Input: dimensioned drawing with shaded views. Units: mm. Origin: part minimum x, y, z. Round coordinates to 2 decimals unless told otherwise and drop trailing zeros. Order: outer loops, then holes, each group sorted by start corner. A loop starts at its lowest first (then second) coordinate and runs counter-clockwise, first axis right, second up. Notation, with made-up numbers: (33.25, 87) - (68.25, 87) arc R31 ccw to (68.25, 122) - close; hole circle Ø3 at (81.5, -8.5). An arc over 180 degrees is marked (long way). Put each result on its own line as item: value. Start each with the question number.
(1) Material intervals for L1, parallel to Y at x = 12, z = 2; L2, parallel to X at y = 38, z = 4.5; L3, parallel to Y at x = 24, z = 2.25, sorted ascending. Write a range as [from, to].
(2) Section C-C (z = 3.35). Output: boundary loops of the cut face in (x, y).
(3) Section A-A (y = 42). Output: boundary loops of the cut face in (x, z), and give its area (3 significant figures).
(4) Section B-B (x = 12). Output: boundary loops of the cut face in (y, z).
(5) Section D-D (x = 84). Output: boundary loops of the cut face in (y, z).
(6) Pin query (flat end, axial travel): P1, Ø1.3, axis at y = 2.5, z = 2, coming from the +X side; P2, Ø3.5, axis at x = 15, y = 74, coming from the +Z side; P3, Ø1.3, axis at y = 78.5, z = 4, coming from the +X side; P4, Ø1, axis at x = 68, z = 1.5, coming from the +Y side. Return the tip coordinate at first contact, or that it passes through.
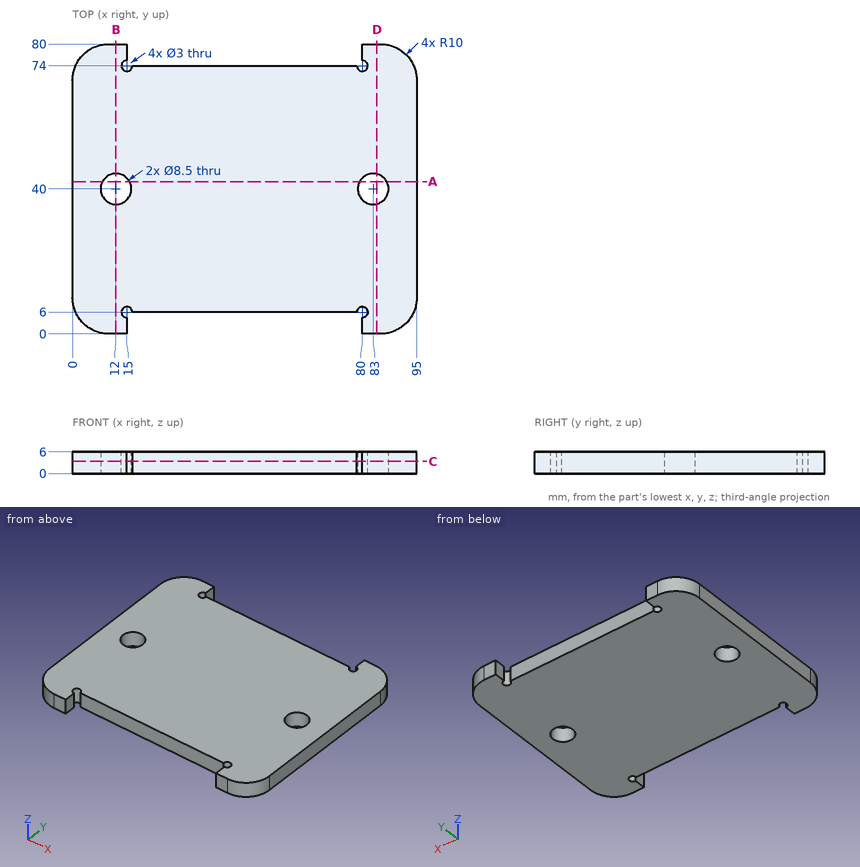
Checks:
1. L1: y = [0, 35.75], [44.25, 80]
1. L2: x = [0, 8.25], [15.75, 79.25], [86.75, 95]
1. L3: y = [6, 74]
2. outline: (0, 10) arc R10 ccw to (10, 0) - (15, 0) - (15, 4.5) arc R1.5 cw (long way) to (16.5, 6) - (78.5, 6) arc R1.5 cw (long way) to (80, 4.5) - (80, 0) - (85, 0) arc R10 ccw to (95, 10) - (95, 70) arc R10 ccw to (85, 80) - (80, 80) - (80, 75.5) arc R1.5 cw (long way) to (78.5, 74) - (16.5, 74) arc R1.5 cw (long way) to (15, 75.5) - (15, 80) - (10, 80) arc R10 ccw to (0, 70) - close; hole circle Ø8.5 at (12, 40); hole circle Ø8.5 at (83, 40)
3. outline: (0, 0) - (8.25, 0) - (8.25, 6) - (0, 6) - close; (15.75, 0) - (79.25, 0) - (79.25, 6) - (15.75, 6) - close; (86.75, 0) - (95, 0) - (95, 6) - (86.75, 6) - close
3. area: 480 mm²
4. outline: (0, 0) - (35.75, 0) - (35.75, 6) - (0, 6) - close; (44.25, 0) - (80, 0) - (80, 6) - (44.25, 6) - close
5. outline: (0, 0) - (35.87, 0) - (35.87, 6) - (0, 6) - close; (44.13, 0) - (80, 0) - (80, 6) - (44.13, 6) - close
6. P1: stops at x = 92.29
6. P2: stops at z = 6
6. P3: stops at x = 91.19
6. P4: stops at y = 74
